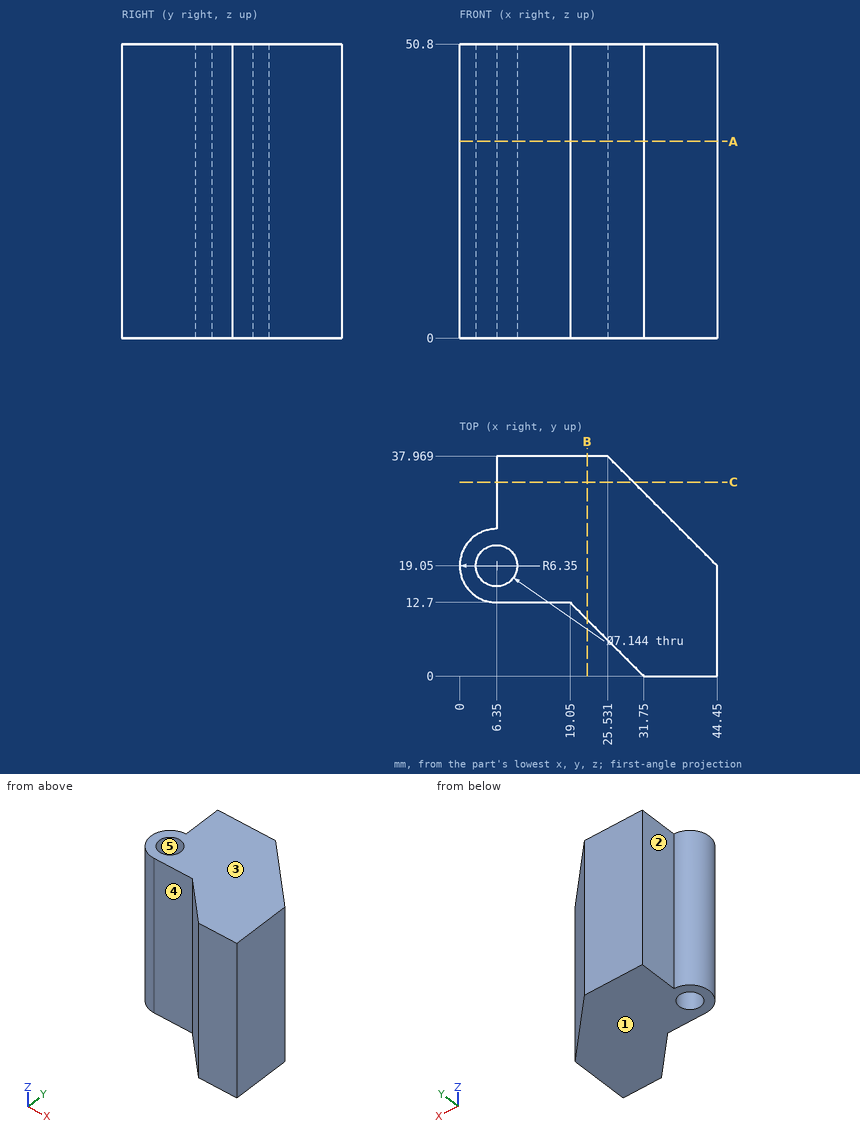
For this review, use the dimensioned drawing (mm, ordinates from the lowest corner) and the shaded views. A direction names the side the tool comes from. Coordinates: 2 decimals unless noted, no trailing zeros. Write each loop counter-clockwise with the first axis right and the second up, starting at its lowest first coordinate (ties: lowest second). Pieces come first, ordered by that corner, then holes. Notation, with made-up numbers: (66, 67) - (123, 67) arc R28 ccw to (123, 102) - close; hole circle Ø10 at (-16, 73.25). An arc over 180 degrees is marked (long way). Answer as a JSON object with one key per item and string values. Group by question number.
1. To check wall thickness, follow probe 1 along X at (y, z) = (19, 15); probe 2 along Y at (x, z) = (6, 15) (1 decimal); probe 3 along X at (y, z) = (22, 46.5) (1 decimal). State the ranges of each line that lie inside material, in increasing order.
2. Clearance check with flat-ended pins moving along their axes: pin 1 Ø6.5 at (x, z) = (10, 17.5) entering from -Y; pin 2 Ø4.5 at (x, y) = (6.35, 19.05) entering from -Z; pin 3 Ø3 at (x, z) = (36, 10.5) entering from -Y; pin 4 Ø4 at (y, z) = (28, 15) entering from +X. State where each tip first meets the part, or that it passes through.
3. Add section B-B (x = 22). Give the boundary of the cut face in (y, z), plus the area to 3 significant figures.
4. Mouldability with a two-part tool opening along Y and no side actions: class the marked faces 3, 4 and 5 as pulls with the +Y half, pulls with the -Y half, needs draft (parallel to the pull), parting line crosses it, or undercut.
5. Add section C-C (y = 33.5). Give the boundary of the cut face in (x, z).
6. Add section A-A (z = 34). Give the boundary of the cut face in (x, y), plus the area to 3 significant figures.
7. Machinability: for the marked faces 1 and 2, which of the approach directions +Z, -Z, +X, -X, +Y, -Y give a long, thin tool a straight path to every point of the face, cutting with its end or side? Answer none if there is none.
Findings:
{
 "1": {"probe 1": "0 to 2.78, 9.92 to 44.45", "probe 2": "12.7 to 15.5, 22.6 to 25.4", "probe 3": "0.7 to 4.3, 8.4 to 41.5"},
 "2": {"pin 1": "y = 12.7", "pin 2": "through", "pin 3": "y = 0", "pin 4": "x = 37.5"},
 "3": {"outline": "(9.75, 0) - (37.97, 0) - (37.97, 50.8) - (9.75, 50.8) - close", "area": "1,430 mm²"},
 "4": {"face 3": "needs draft", "face 4": "pulls with the -Y half", "face 5": "undercut"},
 "5": {"outline": "(6.35, 0) - (30, 0) - (30, 50.8) - (6.35, 50.8) - close"},
 "6": {"outline": "(6.35, 12.7) - (19.05, 12.7) - (31.75, 0) - (44.45, 0) - (44.45, 19.05) - (25.53, 37.97) - (6.35, 37.97) - (6.35, 25.4) arc R6.35 ccw to start; hole circle Ø7.14 at (6.35, 19.05)", "area": "1,050 mm²"},
 "7": {"face 1": "-Z, +X, -X, +Y, -Y", "face 2": "+Z, -Z, -X, +Y"}
}
